Part model, mm, in its own coordinate system. Round coordinates to 2 decimals unless told otherwise and drop trailing zeros. Order: outer loops, then holes, each group sorted by start corner. A loop starts at its lowest first (then second) coordinate and runs counter-clockwise, first axis right, second up. Notation, with made-up numbers: (66, 15) - (85, 15) arc R27 ccw to (85, 50) - close; hole circle Ø1 at (68.25, -11.75). An arc over 180 degrees is marked (long way). Answer as a JSON object with one key per item and string values.
```python
from build123d import *

# Parameters (mm, degrees)
F0_W     = 254
F0_H     = 101.6
F0_R     = 33.310406
F1_DEPTH = 12.7
F2_R     = 5.08
F3_R     = 5.08


with BuildPart() as f1:
    # F0 (on Top) → F1 (new body, symmetric)
    with BuildSketch(Plane.XY):
        Rectangle(F0_W, F0_H)
        Circle(F0_R, mode=Mode.SUBTRACT)
    extrude(amount=F1_DEPTH, both=True)

    # F2
    f2_edges = [f1.edges().sort_by_distance(p)[0] for p in [
        (-33.310406, 0, 12.7),
    ]]
    fillet(f2_edges, radius=F2_R)

    # F3
    f3_edges = [f1.edges().sort_by_distance(p)[0] for p in [
        (0, -50.8, 12.7),
        (0, 50.8, 12.7),
        (-127, 0, 12.7),
        (127, 0, 12.7),
        (127, 50.8, 0),
        (127, 0, -12.7),
        (0, 50.8, -12.7),
        (0, -50.8, -12.7),
        (-33.310406, 0, -12.7),
        (127, -50.8, 0),
        (-127, -50.8, 0),
        (-127, 50.8, 0),
        (-127, 0, -12.7),
    ]]
    fillet(f3_edges, radius=F3_R)


solid = f1.part
```
Item 1: Cut at C-C (y = 0). Write the cut outline in (x, z).
Taken from the geometry:
{"outline": "(-127, -7.62) arc R5.08 ccw to (-121.92, -12.7) - (-38.39, -12.7) arc R5.08 ccw to (-33.31, -7.62) - (-33.31, 7.62) arc R5.08 ccw to (-38.39, 12.7) - (-121.92, 12.7) arc R5.08 ccw to (-127, 7.62) - close; (33.31, -7.62) arc R5.08 ccw to (38.39, -12.7) - (121.92, -12.7) arc R5.08 ccw to (127, -7.62) - (127, 7.62) arc R5.08 ccw to (121.92, 12.7) - (38.39, 12.7) arc R5.08 ccw to (33.31, 7.62) - close"}
Item 2: Two-plate mould, pull along Y, no slides. Class faces 1 (the flat face through (-127, -1, 0)), 2 (the cylindrical face through (1.707, 49.351, -11.172)), 3 (the cylindrical face through (1.707, -49.272, 11.251)), 4 (the cylindrical face through (15.371, -29.552, -0.107)): pulls with the +Y half, pulls with the -Y half, needs draft (parallel to the pull), parting line crosses it, or undercut.
Taken from the geometry:
{"face 1": "needs draft", "face 2": "pulls with the +Y half", "face 3": "pulls with the -Y half", "face 4": "undercut"}
Item 3: Cut at A-A (x = 0). Write the cut outline in (y, z).
Taken from the geometry:
{"outline": "(-50.8, -7.62) arc R5.08 ccw to (-45.72, -12.7) - (-38.39, -12.7) arc R5.08 ccw to (-33.31, -7.62) - (-33.31, 7.62) arc R5.08 ccw to (-38.39, 12.7) - (-45.72, 12.7) arc R5.08 ccw to (-50.8, 7.62) - close; (33.31, -7.62) arc R5.08 ccw to (38.39, -12.7) - (45.72, -12.7) arc R5.08 ccw to (50.8, -7.62) - (50.8, 7.62) arc R5.08 ccw to (45.72, 12.7) - (38.39, 12.7) arc R5.08 ccw to (33.31, 7.62) - close"}
Item 4: Probe L1, parallel to Y at x = 0, z = -4.25; L2, parallel to X at y = -21, z = 2.25; L3, parallel to X at y = 6, z = 10.75. List the from-to ranges inside material, lowest first. Write a range as from..to.
Taken from the geometry:
{"L1": "-50.8..-33.31, 33.31..50.8", "L2": "-127..-25.86, 25.86..127", "L3": "-125.92..-33.86, 33.86..125.92"}
Item 5: Cut at B-B (z = 3). Write the cut outline in (x, y), plus the area to 3 significant figures.
Taken from the geometry:
{"outline": "(-127, -45.72) arc R5.08 ccw to (-121.92, -50.8) - (121.92, -50.8) arc R5.08 ccw to (127, -45.72) - (127, 45.72) arc R5.08 ccw to (121.92, 50.8) - (-121.92, 50.8) arc R5.08 ccw to (-127, 45.72) - close; hole circle Ø66.62 at (0, 0)", "area": "22,300 mm2"}
